from build123d import *

# Parameters (mm, degrees)
SKETCH1_R           = 4.5
BOSS_EXTRUDE1_DEPTH = 1
SKETCH2_R           = 0.5
BOSS_EXTRUDE2_DEPTH = 1
BOSS_EXTRUDE3_DEPTH = 1
BOSS_EXTRUDE4_DEPTH = 1
FILLET1_R           = 1


with BuildPart() as part:
    # Sketch1 → Boss-Extrude1 (new body)
    with BuildSketch(Plane.XY):
        Polygon((4, 6), (4, 8), (-4, 8), (-4, 6), (-7, 6), (-7, 2.5), (-9, 2.5), (-9, -2.5), (-7, -2.5), (-7, -6), (-4, -6), (-4, -8), (4, -8), (4, -6), (7, -6), (7, 6), align=None)
        Circle(SKETCH1_R, mode=Mode.SUBTRACT)
    extrude(amount=BOSS_EXTRUDE1_DEPTH)

    # Sketch2 → Boss-Extrude2 (add)
    with BuildSketch(Plane.ZY.offset(9)):
        with BuildLine():
            Line((1, 2.5), (-1.55, 2.5))
            ThreePointArc((-1.55, 2.5), (-3.282411614, 1.782411614), (-4, 0.05))
            Line((-4, 0.05), (-4, -0.05))
            ThreePointArc((-4, -0.05), (-3.282411614, -1.782411614), (-1.55, -2.5))
            Line((-1.55, -2.5), (1, -2.5))
            Line((1, -2.5), (1, 2.5))
        make_face()
        with Locations((-1.55, -0.05)):
            Circle(SKETCH2_R, mode=Mode.SUBTRACT)
    extrude(amount=BOSS_EXTRUDE2_DEPTH)

    # Sketch3 → Boss-Extrude3 (add)
    with BuildSketch(Plane(origin=(0, 8, 0), x_dir=(1, 0, 0), z_dir=(0, 1, 0))):
        Polygon((4, 0), (4, 16), (7, 16), (7, 19), (-7, 19), (-7, 16), (-4, 16), (-4, 0), (-4, -1), (4, -1), align=None)
    extrude(amount=BOSS_EXTRUDE3_DEPTH)

    # Sketch4 → Boss-Extrude4 (add)
    with BuildSketch(Plane.XZ.offset(8)):
        Polygon((-4, 1), (-4, -16), (-7, -16), (-7, -19), (7, -19), (7, -16), (4, -16), (4, 1), align=None)
    extrude(amount=BOSS_EXTRUDE4_DEPTH)

    # Fillet1
    fillet1_edges = [part.edges().sort_by_distance(p)[0] for p in [
        (-10, 0, 1),
        (0, 9, 1),
        (0, -9, 1),
    ]]
    fillet(fillet1_edges, radius=FILLET1_R)


solid = part.part
Source: CAD feature listing. Evaluate the final solid. Frame: model axes, mm. A direction names the side the tool comes from. Coordinates: 2 decimals unless noted, no trailing zeros. Loops run counter-clockwise (first coordinate to the right, second up) from the corner with the lowest first, then second, coordinate; pieces in that order, holes last. Notation, with made-up numbers: (58, 76.5) - (90, 76.5) arc R15 cw to (90, 92.5) - close; hole circle Ø4 at (-7.75, 41.25). An arc over 180 degrees is marked (long way). One line per item, written item: value. Start each with the question number.
1. Ray query, L1, parallel to Y at x = -1, z = -11.5; L2, parallel to Z at x = -2.75, y = -6.75; L3, parallel to Y at x = -9.3, z = -1.55. Return the intervals inside material, ascending.
2. Section C-C (y = -1.75). Return the cut outline in (x, z).
3. Section B-B (x = 0). Return the cut outline in (y, z), and give its area (3 significant figures).
4. Contact query for flat-ended pins moving along their axis: P1, Ø0.5, axis at x = 6, z = 0.5, coming from the +Y side; P2, Ø2.5, axis at y = -7.5, z = -8, coming from the -X side; P3, Ø2, axis at x = -8.5, z = 0, coming from the -Y side. Output: stop coordinate, or through.
5. Set-up query: faces 4 (the flat face through (5.5, -6, 0.5)), 5 (the flat face through (4, 8.15, -5.49)), 6 (the flat face through (-8.8, -2.5, 0.3)). Return all of +Z, -Z, +X, -X, +Y, -Y with unobstructed straight access to the full face (end or side cutting, diameter ignored); none if empty.
6. Section A-A (z = -7.5). Return the cut outline in (x, y).
7. Mould query, pull axis Y, two halves, no side actions, for faces 1 (the flat face through (-5.5, -8.5, -16)), 2 (the flat face through (5.5, 6, 0.5)), 3 (the flat face through (-5, 0, 0)). Classes: pulls with the +Y half, pulls with the -Y half, needs draft (parallel to the pull), parting line crosses it, or undercut.
8. Section D-D (x = -5.25). Return the cut outline in (y, z), and give its area (3 significant figures).
Verdict:
1. L1: y = -9 to -8, 8 to 9
1. L2: z = 0 to 1
1. L3: y = -2.5 to -0.55, 0.45 to 2.5
2. outline: (-10, -3.31) - (-9, -3.31) - (-9, 0) - (-4.15, 0) - (-4.15, 1) - (-9, 1) arc R1 ccw to (-10, 0) - close; (4.15, 0) - (7, 0) - (7, 1) - (4.15, 1) - close
3. outline: (-9, -19) - (-8, -19) - (-8, 0) - (-4.5, 0) - (-4.5, 1) - (-8, 1) arc R1 ccw to (-9, 0) - close; (4.5, 0) - (8, 0) - (8, -19) - (9, -19) - (9, 0) arc R1 ccw to (8, 1) - (4.5, 1) - close
3. area: 46.6 mm2
4. P1: stops at y = 6
4. P2: stops at x = -4
4. P3: stops at y = -2.5
5. face 4: +Z, -Z, +X, -Y
5. face 5: +Z, +X, +Y
5. face 6: +Z, -Z, -X, -Y
6. outline: (-4, -9) - (4, -9) - (4, -8) - (-4, -8) - close; (-4, 8) - (4, 8) - (4, 9) - (-4, 9) - close
7. face 1: needs draft
7. face 2: pulls with the +Y half
7. face 3: undercut
8. outline: (-9, -19) - (-8, -19) - (-8, -16) - (-9, -16) - close; (-6, 0) - (6, 0) - (6, 1) - (-6, 1) - close; (8, -19) - (9, -19) - (9, -16) - (8, -16) - close
8. area: 18.0 mm2
